```python
from build123d import *

# Parameters (mm, degrees)
ESBO_O1_W                = 90
ESBO_O1_H                = 60
RESSALTO_EXTRUS_O1_DEPTH = 30
CORTE_EXTRUS_O1_DEPTH    = 113.249721603
ESBO_O18_W               = 50
ESBO_O18_H               = 30
CORTE_EXTRUS_O2_DEPTH    = 10
ESBO_O20_R               = 5
CORTE_EXTRUS_O4_DEPTH    = 113.249721603
ESBO_O22_R               = 18
CORTE_EXTRUS_O5_DEPTH    = 5


with BuildPart() as part:
    # Esboço1 → Ressalto-extrusão1 (new body)
    with BuildSketch(Plane(origin=(0, 0, 0), x_dir=(1, 0, 0), z_dir=(0, 1, 0))):
        with Locations((45, 30)):
            Rectangle(ESBO_O1_W, ESBO_O1_H)
    extrude(amount=RESSALTO_EXTRUS_O1_DEPTH)

    # Esboço2 → Corte-extrusão1 (cut, through all)
    with BuildSketch(Plane(origin=(0, 30, 0), x_dir=(1, 0, 0), z_dir=(0, 1, 0))):
        with BuildLine():
            Line((90, 45), (75, 45))
            ThreePointArc((75, 45), (60, 30), (75, 15))
            Line((75, 15), (90, 15))
            Line((90, 15), (90, 45))
        make_face()
    extrude(amount=-CORTE_EXTRUS_O1_DEPTH, mode=Mode.SUBTRACT)

    # Esboço18 → Corte-extrusão2 (cut)
    with BuildSketch(Plane.ZY):
        with Locations((-30, 15)):
            Rectangle(ESBO_O18_W, ESBO_O18_H)
    extrude(amount=-CORTE_EXTRUS_O2_DEPTH, mode=Mode.SUBTRACT)

    # Esboço20 → Corte-extrusão4 (cut, through all)
    with BuildSketch(Plane(origin=(0, 30, 0), x_dir=(1, 0, 0), z_dir=(0, 1, 0))):
        with Locations(Location((35, 30, 0), (0, 0, 270))):
            Circle(ESBO_O20_R)
    extrude(amount=-CORTE_EXTRUS_O4_DEPTH, mode=Mode.SUBTRACT)

    # Esboço22 → Corte-extrusão5 (cut)
    with BuildSketch(Plane(origin=(0, 30, 0), x_dir=(1, 0, 0), z_dir=(0, 1, 0))):
        with Locations(Location((35, 30, 0), (0, 0, 270))):
            Circle(ESBO_O22_R)
    extrude(amount=-CORTE_EXTRUS_O5_DEPTH, mode=Mode.SUBTRACT)


solid = part.part
```
Geometry check sheet. Reference: the model listing, model coordinates, mm. A direction names the side the tool comes from. Coordinates: 2 decimals unless noted, no trailing zeros. Write each loop counter-clockwise with the first axis right and the second up, starting at its lowest first coordinate (ties: lowest second). Pieces come first, ordered by that corner, then holes. Notation, with made-up numbers: M 22.5,-37 L 70.5,-37 A28 ccw 70.5,-19 Z; hole C -26.75,23 d2. An arc over 180 degrees is marked long. Use one line per item in the form item = value. Start each with the question number.
1) Release check for a two-part mould opening along Z. For faces 1 (the flat face through (5, 15, -55)), 2 (the flat face through (44, 15, 0)), 3 (the cylindrical face through (60, 15, -30)), 4 (the flat face through (54, 30, -30)) record: pulls with the +Z half, pulls with the -Z half, needs draft (parallel to the pull), parting line crosses it, or undercut.
2) Section check A-A on y = 14.5. Enter the section's corners in (x, z).
3) Section check C-C on x = 81. Enter the section's corners in (y, z), and give its area (3 significant figures).
4) Section check B-B on z = -30. Enter the section's corners in (x, y).
5) Set-up check for faces 5 (the flat face through (5, 15, -5)), 6 (the flat face through (82, 15, -15)), 7 (the cylindrical face through (40.407, 27.535, -12.831)): record each of +Z, -Z, +X, -X, +Y, -Y from which the full face is reachable in a straight line by a thin tool's end or side.
6) Go/stop test with flat-tipped pins: pin 1 Ø1 at (y, z) = (26.5, -32) entering from -X; pin 2 Ø13 at (x, z) = (35, -30) entering from +Y; pin 3 Ø1 at (y, z) = (21, -25.5) entering from +X. Record where each tip stops, or that it passes through.
7) Thickness scan on probe 1 along Z at (x, y) = (76, 2); probe 2 along Z at (x, y) = (7.5, 2); probe 3 along X at (y, z) = (11.75, -30). Record the ranges inside material, lowest first. Write a range as from..to.
8) Section check D-D on z = -40. Enter the section's corners in (x, y), and give its area (3 significant figures).
Responses:
q1.face_1 = undercut
q1.face_2 = pulls with the +Z half
q1.face_3 = undercut
q1.face_4 = needs draft
q2.outline = M 0,-60 L 90,-60 L 90,-45 L 75,-45 A15 cw 75,-15 L 90,-15 L 90,0 L 0,0 L 0,-5 L 10,-5 L 10,-55 L 0,-55 Z; hole C 35,-30 d10
q3.outline = M 0,-60 L 30,-60 L 30,-45 L 0,-45 Z; M 0,-15 L 30,-15 L 30,0 L 0,0 Z
q3.area = 900 mm2
q4.outline = M 10,0 L 30,0 L 30,25 L 17,25 L 17,30 L 10,30 Z; M 40,0 L 60,0 L 60,30 L 53,30 L 53,25 L 40,25 Z
q5.face_5 = -X, +Y, -Y
q5.face_6 = +X, +Y, -Y
q5.face_7 = +Y
q6.pin_1 = 10
q6.pin_2 = 25
q6.pin_3 = 60.86
q7.probe_1 = -60..-45, -15..0
q7.probe_2 = -60..-55, -5..0
q7.probe_3 = 10..30, 40..60
q8.outline = M 10,0 L 63.82,0 L 63.82,30 L 49.97,30 L 49.97,25 L 20.03,25 L 20.03,30 L 10,30 Z
q8.area = 1,460 mm2
